from build123d import *

# Parameters (mm, degrees)
SKETCH_2_R      = 5
SKETCH_2_R_2    = 7.5
EXTRUDE_1_DEPTH = 5
FILLET_1_R      = 200
FILLET_2_R      = 100
FILLET_3_R      = 15


with BuildPart() as part:
    # 草图2 → 凸台-拉伸1 (new body)
    with BuildSketch(Plane.XY):
        with BuildLine():
            Line((-152.644904711, 15), (-249.099564228, -20.106625021))
            ThreePointArc((-249.099564228, -20.106625021), (-258.06465139, -39.332316482), (-238.838959929, -48.297403644))
            Line((-238.838959929, -48.297403644), (-147.355095289, -15))
            Line((-147.355095289, -15), (13.989229745, -15))
            Line((13.989229745, -15), (67.976465972, 49.339482728))
            Line((67.976465972, 49.339482728), (44.995132678, 68.623111018))
            Line((44.995132678, 68.623111018), (0, 15))
            Line((0, 15), (-152.644904711, 15))
        make_face()
        with Locations((0, 5)):
            Circle(SKETCH_2_R, mode=Mode.SUBTRACT)
        with Locations((17.699325905, 14.313101658)):
            Circle(SKETCH_2_R_2, mode=Mode.SUBTRACT)
    extrude(amount=EXTRUDE_1_DEPTH)

    # 圆角1
    fillet_1_edges = [part.edges().sort_by_distance(p)[0] for p in [
        (-152.644904711, 15, 2.5),
        (-147.355095289, -15, 2.5),
    ]]
    fillet(fillet_1_edges, radius=FILLET_1_R)

    # 圆角2
    fillet_2_edges = [part.edges().sort_by_distance(p)[0] for p in [
        (0, 15, 2.5),
        (13.989229745, -15, 2.5),
    ]]
    fillet(fillet_2_edges, radius=FILLET_2_R)

    # 圆角3
    fillet_3_edges = [part.edges().sort_by_distance(p)[0] for p in [
        (44.995132678, 68.623111018, 2.5),
        (67.976465972, 49.339482728, 2.5),
    ]]
    fillet(fillet_3_edges, radius=FILLET_3_R - 0.0001)  # a hair under: the kernel refuses the full size


solid = part.part
Build history of the part. All positions in model axes, mm. Give positions to 0.01 mm unless a question says otherwise; leave off trailing zeros. Order: outer loops, then holes, each group sorted by start corner. A loop starts at its lowest first (then second) coordinate and runs counter-clockwise, first axis right, second up. Notation, with made-up numbers: M -26.5,8.25 L 24.5,8.25 A18 ccw 24.5,28.25 Z; hole C 39,85.5 d2. An arc over 180 degrees is marked long. Use one line per item in the form item = value.
Q1. Slice it at C-C, the plane x = -49.5. Write the cut outline in (y, z).
Conclusion:
outline = M -15,0 L 15,0 L 15,5 L -15,5 Z
Q2. Wall check: probe 1 along Y at (x, z) = (-112, 1.8); probe 2 along Y at (x, z) = (17, 1.15); probe 3 along Y at (x, z) = (-32.5, 2.8). Give the ranges that are in metal, low to high.
Conclusion:
probe_1 = -15 to 15
probe_2 = -1.81 to 6.85, 21.78 to 37.86
probe_3 = -15 to 16
Q3. Pull direction Y, two halves, no side cores. Call faces 1 (the cylindrical face through (-4.923, 24.113, 2.535)), 2 (the flat face through (51.05, 29.17, 2.46)), 3 (the cylindrical face through (12.17, 19.38, 2.46)), 4 (the flat face through (-99, -1, 0)): released by +Y, released by -Y, zero draft, split by the parting line, or undercut.
Conclusion:
face_1 = released by +Y
face_2 = released by -Y
face_3 = undercut
face_4 = zero draft
Q4. Slice it at A-A, the plane x = 0. Write the cut outline in (y, z), and give its area (3 significant figures).
Conclusion:
outline = M -9.52,0 L 0,0 L 0,5 L -9.52,5 Z; M 10,0 L 26.54,0 L 26.54,5 L 10,5 Z
area = 130 mm2
Q5. Pin check, flat tips, straight feed: P1, Ø2.5, axis at x = -70, z = 2, coming from the -Y side; P2, Ø8, axis at x = 0, y = 5, coming from the +Z side; P3, Ø3, axis at x = 0, z = 1, coming from the +Y side. Stop position of each tip, or through.
Conclusion:
P1 = -15
P2 = through
P3 = 27.34
Q6. Slice it at D-D, the plane y = -38.5. Write the cut outline in (x, z), and give its area (3 significant figures).
Conclusion:
outline = M -258.34,0 L -211.92,0 L -211.92,5 L -258.34,5 Z
area = 232 mm2
Q7. Slice it at B-B, the plane z = 2.5. State how many separate pieces and enclosed holes the cut face has, and give its area (3 significant figures).
Conclusion:
separate_pieces = 1
enclosed_holes = 2
area = 10,000 mm2
